Input: part model. Units: mm. Frame: model coordinates. Face numbers are marked on the shaded views. A direction names the side the tool comes from. Coordinates: 2 decimals unless noted, no trailing zeros. Write each loop counter-clockwise with the first axis right and the second up, starting at its lowest first coordinate (ties: lowest second). Pieces come first, ordered by that corner, then holes. Notation, with made-up numbers: M 58.5,29.25 L 62.5,29.25 A9 cw 62.5,44.25 Z; hole C 34.25,-32.75 d5. An arc over 180 degrees is marked long. Use one line per item in the form item = value.
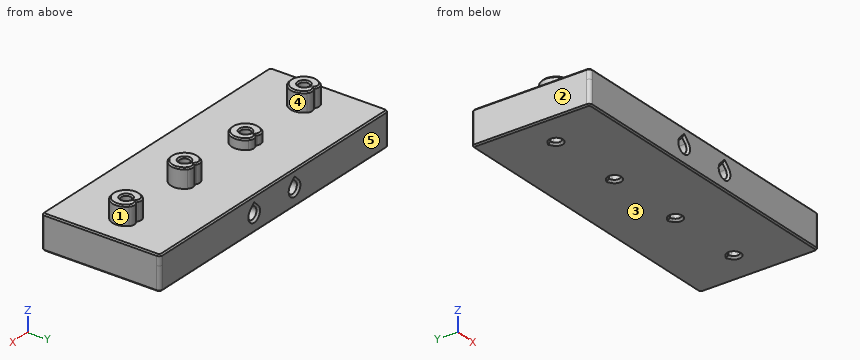
from build123d import *

# Parameters (mm, degrees)
SKETCH_W                = 90
SKETCH_H                = 35
PAD_DEPTH               = 3
SKETCH001_R             = 10.5
HOLE_DEPTH              = 25
HOLE_TEARDROPS_DEPTH    = 25
SKETCH002_R             = 4
PAD001_DEPTH            = 5.6
POCKET_DEPTH            = 5.6
SKETCH004_R             = 1.45
HOLE001_DEPTH           = 25
HOLE001_TEARDROPS_DEPTH = 25
FILLET_R                = 2
CHAMFER_SIZE            = 0.4
FILLET001_R             = 1
PAD002_DEPTH            = 7
SKETCH005_R             = 14.71653
PAD003_DEPTH            = 10
SKETCH006_R             = 4.05
PAD004_DEPTH            = 3
POCKET001_DEPTH         = 3
SKETCH008_R             = 1.45
HOLE002_DEPTH           = 25
HOLE002_TEARDROPS_DEPTH = 25
FILLET002_R             = 2
CHAMFER001_SIZE         = 0.4
CHAMFER002_SIZE         = 0.4
CHAMFER003_SIZE         = 0.6
SKETCH009_R             = 1.7
HOLE003_DEPTH           = 87
HOLE003_TEARDROPS_DEPTH = 87
CHAMFER004_SIZE         = 0.6


with BuildPart() as part:
    # Sketch → Pad (new body)
    with BuildSketch(Plane.XY):
        Rectangle(SKETCH_W, SKETCH_H)
    extrude(amount=PAD_DEPTH)

    # Sketch001 (on Face6 of Pad) → Hole (cut)
    with BuildSketch(Plane.XY.offset(3)):
        with Locations((-12, 0)):
            Circle(SKETCH001_R)
    extrude(amount=-HOLE_DEPTH, mode=Mode.SUBTRACT)

    # Sketch001_Teardrops (on Sketch) → Hole_Teardrops (cut)
    with BuildSketch(Plane.XY.offset(3)):
        with BuildLine():
            ThreePointArc((-17.25, 9.093267), (-12, -10.5), (-6.75, 9.093267))
            Line((-6.75, 9.093267), (-12, 12.124356))
            Line((-17.25, 9.093267), (-12, 12.124356))
        make_face()
    extrude(amount=-HOLE_TEARDROPS_DEPTH, mode=Mode.SUBTRACT)

    # Sketch002 (on Face5 of Hole_Teardrops) → Pad001 (join)
    with BuildSketch(Plane.XY.offset(3)):
        with Locations((35, 0)):
            Circle(SKETCH002_R)
        with Locations((12, 0)):
            Circle(SKETCH002_R)
        with Locations((-35, 0)):
            Circle(SKETCH002_R)
    extrude(amount=PAD001_DEPTH)

    # Sketch003 (on Face13 of Pad001) → Pocket (cut)
    with BuildSketch(Plane.XY.offset(8.6)):
        Polygon((-35, 3), (-38.464102, 5), (-31.535898, 5), align=None)
        Polygon((12, 3), (8.535898, 5), (15.464102, 5), align=None)
        Polygon((38.464102, 5), (35, 3), (31.535898, 5), align=None)
    extrude(amount=-POCKET_DEPTH, mode=Mode.SUBTRACT)

    # Sketch004 (on Face17 of Pocket) → Hole001 (cut)
    with BuildSketch(Plane.XY.offset(8.6)):
        with Locations((-35, 0)):
            Circle(SKETCH004_R)
        with Locations((12, 0)):
            Circle(SKETCH004_R)
        with Locations((35, 0)):
            Circle(SKETCH004_R)
    extrude(amount=-HOLE001_DEPTH, mode=Mode.SUBTRACT)

    # Sketch004_Teardrops (on Sketch) → Hole001_Teardrops (cut)
    with BuildSketch(Plane.XY.offset(8.6)):
        with BuildLine():
            ThreePointArc((-35.725, 1.255737), (-35, -1.45), (-34.275, 1.255737))
            Line((-34.275, 1.255737), (-35, 1.674316))
            Line((-35.725, 1.255737), (-35, 1.674316))
        make_face()
        with BuildLine():
            ThreePointArc((11.275, 1.255737), (12, -1.45), (12.725, 1.255737))
            Line((12.725, 1.255737), (12, 1.674316))
            Line((11.275, 1.255737), (12, 1.674316))
        make_face()
        with BuildLine():
            ThreePointArc((34.275, 1.255737), (35, -1.45), (35.725, 1.255737))
            Line((35.725, 1.255737), (35, 1.674316))
            Line((34.275, 1.255737), (35, 1.674316))
        make_face()
    extrude(amount=-HOLE001_TEARDROPS_DEPTH, mode=Mode.SUBTRACT)

    # Fillet
    fillet_edges = [part.edges().sort_by_distance(p)[0] for p in [
        (36.334875, 3.770691, 5.8),
        (33.665125, 3.770691, 5.8),
        (13.334875, 3.770691, 5.8),
        (10.665125, 3.770691, 5.8),
        (-33.665125, 3.770691, 5.8),
        (-36.334875, 3.770691, 5.8),
    ]]
    fillet(fillet_edges, radius=FILLET_R)

    # Chamfer
    chamfer_edges = [part.edges().sort_by_distance(p)[0] for p in [
        (33.392214, -3.662653, 8.6),
        (10.392214, -3.662653, 8.6),
        (-36.607786, -3.662653, 8.6),
        (-35.725, -1.255737, 8.6),
        (11.275, -1.255737, 8.6),
        (34.275, -1.255737, 8.6),
    ]]
    chamfer(chamfer_edges, length=CHAMFER_SIZE)

    # Fillet001
    fillet001_edges = [part.edges().sort_by_distance(p)[0] for p in [
        (45, 17.5, 1.5),
        (-45, 17.5, 1.5),
        (-45, -17.5, 1.5),
        (45, -17.5, 1.5),
    ]]
    fillet(fillet001_edges, radius=FILLET001_R)

    # Fillet001 Face28 → Pad002 (add)
    with BuildSketch(Plane(origin=(1.493435, -0.023344, 0), x_dir=(0, -1, 0), z_dir=(0, 0, -1))):
        with BuildLine():
            Line((16.476656, 46.493435), (-16.523344, 46.493435))
            ThreePointArc((-16.523344, 46.493435), (-17.230451, 46.200542), (-17.523344, 45.493435))
            Line((-17.523344, 45.493435), (-17.523344, -42.506565))
            ThreePointArc((-17.523344, -42.506565), (-17.230451, -43.213672), (-16.523344, -43.506565))
            Line((-16.523344, -43.506565), (16.476656, -43.506565))
            ThreePointArc((16.476656, -43.506565), (17.183762, -43.213672), (17.476656, -42.506565))
            Line((17.476656, -42.506565), (17.476656, 45.493435))
            ThreePointArc((17.476656, 45.493435), (17.183762, 46.200542), (16.476656, 46.493435))
        make_face()
        with BuildLine():
            ThreePointArc((-0.023344, 35.043435), (-0.748344, 35.237698), (-1.279081, 35.768435))
            Line((-1.279081, 35.768435), (-1.69766, 36.493435))
            Line((-1.69766, 36.493435), (-1.279081, 37.218435))
            ThreePointArc((-1.279081, 37.218435), (1.232392, 37.218435), (-0.023344, 35.043435))
        make_face(mode=Mode.SUBTRACT)
        with BuildLine():
            ThreePointArc((-0.023344, -11.956565), (-0.748344, -11.762302), (-1.279081, -11.231565))
            Line((-1.279081, -11.231565), (-1.69766, -10.506565))
            Line((-1.69766, -10.506565), (-1.279081, -9.781565))
            ThreePointArc((-1.279081, -9.781565), (1.232392, -9.781565), (-0.023344, -11.956565))
        make_face(mode=Mode.SUBTRACT)
        with BuildLine():
            ThreePointArc((-0.023344, -34.956565), (-0.748344, -34.762302), (-1.279081, -34.231565))
            Line((-1.279081, -34.231565), (-1.69766, -33.506565))
            Line((-1.69766, -33.506565), (-1.279081, -32.781565))
            ThreePointArc((-1.279081, -32.781565), (1.232392, -32.781565), (-0.023344, -34.956565))
        make_face(mode=Mode.SUBTRACT)
        with BuildLine():
            ThreePointArc((-0.023344, 2.993435), (-5.273344, 4.400168), (-9.116611, 8.243435))
            Line((-9.116611, 8.243435), (-12.1477, 13.493435))
            Line((-12.1477, 13.493435), (-9.116611, 18.743435))
            ThreePointArc((-9.116611, 18.743435), (9.069922, 18.743435), (-0.023344, 2.993435))
        make_face(mode=Mode.SUBTRACT)
    extrude(amount=PAD002_DEPTH)

    # Sketch005 (on Face3 of Pad002) → Pad003 (join)
    with BuildSketch(Plane.XY.offset(3)):
        with Locations((-11.639154, 0)):
            Circle(SKETCH005_R)
    extrude(amount=-PAD003_DEPTH)

    # Sketch006 (on Face67 of Pad003) → Pad004 (join)
    with BuildSketch(Plane.XY.offset(3)):
        with Locations((-12, 0)):
            Circle(SKETCH006_R)
    extrude(amount=PAD004_DEPTH)

    # Sketch007 (on Face66 of Pad004) → Pocket001 (cut)
    with BuildSketch(Plane.XY.offset(6)):
        Polygon((-12, 3), (-15.464102, 5), (-8.535898, 5), align=None)
    extrude(amount=-POCKET001_DEPTH, mode=Mode.SUBTRACT)

    # Sketch008 (on Face69 of Pocket001) → Hole002 (cut)
    with BuildSketch(Plane.XY.offset(6)):
        with Locations((-12, 0)):
            Circle(SKETCH008_R)
    extrude(amount=-HOLE002_DEPTH, mode=Mode.SUBTRACT)

    # Sketch008_Teardrops (on Sketch) → Hole002_Teardrops (cut)
    with BuildSketch(Plane.XY.offset(6)):
        with BuildLine():
            ThreePointArc((-12.725, 1.255737), (-12, -1.45), (-11.275, 1.255737))
            Line((-11.275, 1.255737), (-12, 1.674316))
            Line((-12.725, 1.255737), (-12, 1.674316))
        make_face()
    extrude(amount=-HOLE002_TEARDROPS_DEPTH, mode=Mode.SUBTRACT)

    # Fillet002
    fillet002_edges = [part.edges().sort_by_distance(p)[0] for p in [
        (-10.608429, 3.803424, 4.5),
        (-13.391571, 3.803424, 4.5),
    ]]
    fillet(fillet002_edges, radius=FILLET002_R)

    # Chamfer001
    chamfer001_edges = [part.edges().sort_by_distance(p)[0] for p in [
        (-12.725, -1.255737, 6),
        (-13.613716, -3.714623, 6),
    ]]
    chamfer(chamfer001_edges, length=CHAMFER001_SIZE)

    # Chamfer002
    chamfer002_edges = [part.edges().sort_by_distance(p)[0] for p in [
        (0, -17.5, -7),
        (0, -17.5, 3),
    ]]
    chamfer(chamfer002_edges, length=CHAMFER002_SIZE)

    # Chamfer003
    chamfer003_edges = [part.edges().sort_by_distance(p)[0] for p in [
        (11.275, -1.255737, -7),
        (34.275, -1.255737, -7),
        (-12.725, -1.255737, -7),
        (-35.725, -1.255737, -7),
    ]]
    chamfer(chamfer003_edges, length=CHAMFER003_SIZE)

    # Sketch009 (on Face29 of Chamfer003) → Hole003 (cut)
    with BuildSketch(Plane.XZ.offset(17.5)):
        with Locations((-7.95, -2)):
            Circle(SKETCH009_R)
        with Locations((7.95, -2)):
            Circle(SKETCH009_R)
    extrude(amount=-HOLE003_DEPTH, mode=Mode.SUBTRACT)

    # Sketch009_Teardrops (on Sketch) → Hole003_Teardrops (cut)
    with BuildSketch(Plane.XZ.offset(17.5)):
        with BuildLine():
            ThreePointArc((-9.152082, -0.797918), (-7.95, -3.7), (-6.747918, -0.797918))
            Line((-6.747918, -0.797918), (-7.95, 0.404163))
            Line((-9.152082, -0.797918), (-7.95, 0.404163))
        make_face()
        with BuildLine():
            ThreePointArc((6.747918, -0.797918), (7.95, -3.7), (9.152082, -0.797918))
            Line((9.152082, -0.797918), (7.95, 0.404163))
            Line((6.747918, -0.797918), (7.95, 0.404163))
        make_face()
    extrude(amount=-HOLE003_TEARDROPS_DEPTH, mode=Mode.SUBTRACT)

    # Chamfer004
    chamfer004_edges = [part.edges().sort_by_distance(p)[0] for p in [
        (-7.299438, -17.5, -3.570595),
        (8.600562, -17.5, -3.570595),
        (-7.299438, 17.5, -3.570595),
        (8.600562, 17.5, -3.570595),
    ]]
    chamfer(chamfer004_edges, length=CHAMFER004_SIZE)


solid = part.part
(1) Set-up query: the marked faces 4 and 5. Return all of +Z, -Z, +X, -X, +Y, -Y with unobstructed straight access to the full face (end or side cutting, diameter ignored); none if empty.
Computed:
face_4 = +Z
face_5 = +Z, -Z, +X, -X, +Y
(2) Section query C-C on x = -28. Return the cut outline in (y, z).
Computed:
outline = M -17.5,-6.6 L -17.1,-7 L 17.1,-7 L 17.5,-6.6 L 17.5,2.6 L 17.1,3 L -17.1,3 L -17.5,2.6 Z
(3) First-contact query: pin 1 Ø3.5 at (x, y) = (-12, 1.5) entering from +Z; pin 2 Ø4 at (x, y) = (12, 0) entering from -Z; pin 3 Ø4.5 at (x, z) = (-7.95, -2) entering from +Y. Flat tips, straight axial feed; report the tip coordinate or a pass-through.
Computed:
pin_1 = 6
pin_2 = -6.95
pin_3 = 17.45
(4) Section query A-A on y = 7. Return the cut outline in (x, z).
Computed:
outline = M -45,-6.6 L -44.6,-7 L 44.6,-7 L 45,-6.6 L 45,2.6 L 44.6,3 L -44.6,3 L -45,2.6 Z; hole M -9.15,-0.8 A1.7 ccw long -6.75,-0.8 L -7.95,0.4 Z; hole M 6.75,-0.8 A1.7 ccw long 9.15,-0.8 L 7.95,0.4 Z
(5) Pull-direction query (X, two-part tool) for the marked faces 1, 2 and 3; classes: pulls with the +X half, pulls with the -X half, needs draft (parallel to the pull), parting line crosses it, or undercut.
Computed:
face_1 = undercut
face_2 = pulls with the -X half
face_3 = needs draft
(6) Line query: probe 1 along Y at (x, z) = (12, -4.25); probe 2 along X at (y, z) = (-3, -1.25); probe 3 along Z at (x, y) = (-12, 7.5). Output: solid intervals per line, ascending.
Computed:
probe_1 = -17.5 to -1.45, 1.67 to 17.5
probe_2 = -45 to -9.48, -6.42 to 6.42, 9.48 to 45
probe_3 = -7 to 3
(7) Section query B-B on z = -2. State how many separate pieces and enclosed holes the cut face has, plus the area to 3 significant figures.
Computed:
separate_pieces = 3
enclosed_holes = 4
area = 2,880 mm^2
